Part model, mm, in its own coordinate system. A direction names the side the tool comes from. Round coordinates to 2 decimals unless told otherwise and drop trailing zeros. Write each loop counter-clockwise with the first axis right and the second up, starting at its lowest first coordinate (ties: lowest second). Pieces come first, ordered by that corner, then holes.
1) Which spindle directions (+Z, -Z, +X, -X, +Y, -Y) get a long thin tool onto all of the face, cutting with end or side? Do faces 1 (the flat face through (-7.359, -2.028, -3.448)), 2 (the flat face through (45, 0, 0)). Say none if no direction does.
2) Drill centre lines: L1, parallel to X at y = 1.5, z = 6; L2, parallel to Y at x = 38, z = 3. Where is each one in solid material? Low to high.
3) Flat gauge pins, fed straight in: pin 1 (1 mm diameter, centred on x = 27.5, y = -3.5, fed in from +Z); pin 2 (2 mm diameter, centred on x = 7, y = 2, fed in from -Z); pin 3 (3 mm diameter, centred on x = 38, y = 0, fed in from +Z). Where does each tip first touch, or does it go through?
4) Pull direction Y, two halves, no side cores. Call faces 3 (the conical face through (-2.5, 0.276, -0.087)), 4 (the cylindrical face through (21.78, -1.08, 4.88)), 5 (the flat face through (0, 5, -2)): +Y half, -Y half, draft (parallel to the pull), parting line (faces both ways), or undercut.
5) Saw through at A-A on x = 9.5. Write the cut outline in (y, z).
Autodesk Inventor part; units mm, degrees
ref_plane "Work Plane1" through (29, 0, 0) normal (0, -1, 0) x (1, 0, 0)
ref_plane "YZ Plane" through (0, 0, 0) normal (1, 0, 0) x (0, 1, 0)
ref_plane "XZ Plane" through (0, 0, 0) normal (0, 1, 0) x (-1, 0, 0)
sketch "Sketch1" plane through (0, 0, 0) normal (0, 0, 1) x (1, 0, 0)
  line L0 (-2.3333, 0) -> (45, 0)
  line L1 (45, 0) -> (45, 5)
  line L2 (45, 5) -> (13, 5)
  line L3 (13, 5) -> (12.0797, 5)
  line L4 (12.0797, 5) -> (0, 5)
  line L5 (0, 5) -> (0, 8)
  line L6 (0, 8) -> (-10, 8)
  line L7 (-10, 8) -> (-10, 4.6188)
  line L8 (-10, 4.6188) -> (-5, 4.6188)
  line L9 (-5, 4.6188) -> (-2.3333, 0)
  line L10 (-21, 0) -> (56, 0)
  line L11 (0, -1.6) -> (0, 9.6)
  line L12 (13, 5) -> (0, 5) construction
  dimension "d1" = 32
  dimension "d2" = 0.9203
  dimension "d3" = 10
  dimension "d4" = 5
  dimension "d5" = 60
  dimension "d6" = 10
  dimension "d7" = 10
  dimension "d8" = 9.2376
  dimension "d9" = 16
  dimension "d26" = 45
revolve "Body" add sketch "Sketch1" angle 360 about axis through (-2.3333, 0, 0) along (1, 0, 0)
sketch "Sketch2" plane through (-10, 0, 0) normal (-1, 0, 0) x (0, 0, 1)
  circle A0 centre (0, 0) radius 4.6188
  line L0 (0, -11.2) -> (0, 11.2)
  line L1 (-11.2, 0) -> (11.2, 0)
  line L2 (4.6188, 0) -> (2.3094, -4)
  line L3 (2.3094, -4) -> (-2.3094, -4)
  line L4 (-2.3094, -4) -> (-4.6188, 0)
  line L5 (-4.6188, 0) -> (-2.3094, 4)
  line L6 (-2.3094, 4) -> (2.3094, 4)
  line L7 (2.3094, 4) -> (4.6188, 0)
extrude "Slot" add sketch "Sketch2" against normal up to next contours L7 A0 | A0 L2 | L6 L0 A0 | A0 L0 L3 | L0 L6 A0 | A0 L3 L0 | L4 A0 | A0 L5
fillet "Fillet1" radius 1 1 edges at (-10, -8, 0)
thread "Thread"
chamfer "Chamfer1" distance 0.9202 distance2 0.9202 1 edges at (45, -5, 0) measured on face at (45, -1.105, 0.7295)
ref_plane "Work Plane1" through (29, 0, 0) normal (0, -1, 0) x (1, 0, 0)
fillet "Fillet2" radius 0.1 1 edges at (0, -5, 0)
equation "\"d1\" = GEL"
equation "\"d3\" = KOH"
equation "\"d4\" = INTI"
equation "\"d6\" = GD"
equation "\"d7\" = BDM"
equation "\"d8\" = 1.1547 * SW"
equation "\"d9\" = KOD"
equation "\"d26\" = NLG"
equation "\"d30\" = R"
equation "\"d17\" = RR"
equation "\"d13\" = GEL"
equation "\"d15\" = -0.5 * SPD + 0.5 * GD"
equation "\"d16\" = GUL"
equation "\"GD\" = NND"
equation "\"NLG\" = 45"
equation "\"GEL\" = 32"
equation "\"KOD\" = 16"
equation "\"KOH\" = NND"
equation "\"INTI\" = 5"
equation "\"GAL\" = 0.61345 * PTC"
equation "\"GUL\" = 0.61345 * PTC"
equation "\"BDM\" = NND"
equation "\"SW\" = 8"
equation "\"RR\" = 0.1 * NND"
equation "\"SPD\" = NND - 1.2269 * PTC"
equation "\"R\" = 0.1"
equation "\"TOA\" = 30deg"
equation "\"GD1\" = THREADDIA - 1.2269 * PTC"
equation "\"FAWI\" = 45deg"
equation "\"PTC\" = 1.5"
equation "\"E0\" = 1.155 * SW"
properties part number "M10x35 SHCS A2" material "Stainless Steel AISI 304"
Completed:
1. face 1: -X
1. face 2: +Z, -Z, +X, +Y, -Y
2. L1: x = -10 to 0
2. L2: y = -4 to 4
3. pin 1: stops at z = 4
3. pin 2: stops at z = -4.9
3. pin 3: stops at z = 5
4. face 3: undercut
4. face 4: parting line
4. face 5: draft
5. outline: circle Ø10 at (0, 0)
